Study the drawing (mm; zero at the part's minimum x, y, z) and answer. A direction names the side the tool comes from. Round coordinates to 2 decimals unless told otherwise and drop trailing zeros. Order: outer loops, then holes, each group sorted by start corner. A loop starts at its lowest first (then second) coordinate and runs counter-clockwise, first axis right, second up. Notation, with made-up numbers: (23.25, 50.25) - (46.25, 50.25) arc R23 cw to (46.25, 73.25) - close; hole circle Ø11 at (13, 67). An arc over 180 degrees is marked (long way). Put each result on its own line as item: value. Start each with the question number.
Q1. Each of these flat-tipped pins is pushed along its axis until it touches: pin 1 Ø3 at (x, z) = (9, 3) entering from +Y; pin 2 Ø3 at (x, z) = (13, 9.5) entering from -Y; pin 3 Ø1.5 at (y, z) = (1, 12.5) entering from -X; pin 4 Ø0.8 at (x, z) = (19.5, 18) entering from +Y. Where does it stop, or does it pass through?
Q2. Find the intervals of material crossed by line 1 along X through (y, z) = (6.9, 17.5) (3 decimals); line 2 along Z through (x, y) = (13.5, 3); line 3 along Y through (x, z) = (11, 12.5), in increasing order. Write a range as from..to.
Q3. Section C-C on z = 17.5 is taken. Give the vertices of the cut face in (x, y) (3 decimals), then the cut area to 3 significant figures.
Q4. Which of the six approach directions +Z, -Z, +X, -X, +Y, -Y give full straight-line access (tool end or side, diameter ignored) to the marked faces 5 and 6?
Q5. For a pull along Z with two mould halves and no side action, classify the marked faces 1, 2, 3 and 4 as pulls with the +Z half, pulls with the -Z half, needs draft (parallel to the pull), parting line crosses it, or undercut.
Q6. Section A-A on x = 19.45 is taken. Give the vertices of the cut face in (y, z) (3 decimals).
Q7. Section B-B on y = 4 is taken. Give the vertices of the cut face in (x, z).
Q8. Section D-D on x = 24.5 is taken. Give the vertices of the cut face in (y, z).
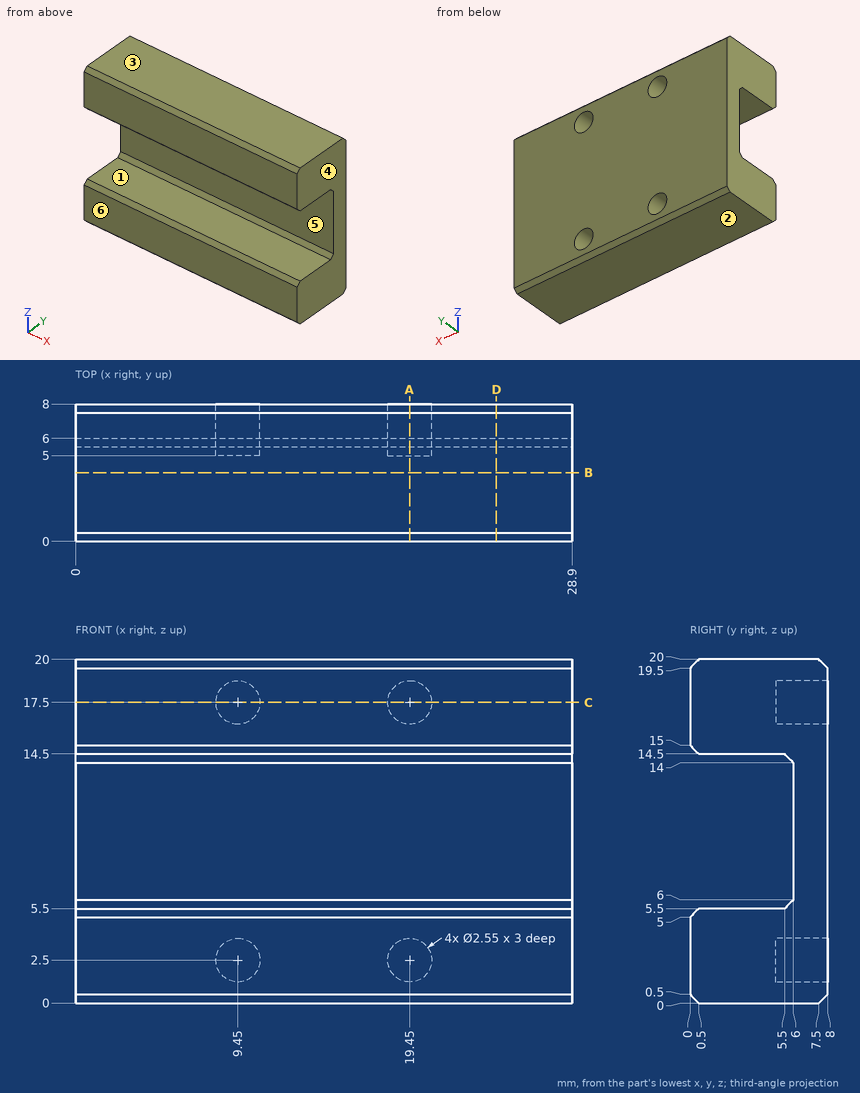
Findings:
1. pin 1: y = 8
1. pin 2: y = 6
1. pin 3: through
1. pin 4: y = 5
2. line 1: 0..8.175, 10.725..18.175, 20.725..28.9
2. line 2: 0..5.5, 14.5..20
2. line 3: 6..8
3. outline: (0, 0) - (28.9, 0) - (28.9, 8) - (20.725, 8) - (20.725, 5) - (18.175, 5) - (18.175, 8) - (10.725, 8) - (10.725, 5) - (8.175, 5) - (8.175, 8) - (0, 8) - close
3. area: 216 mm2
4. face 5: +X, -X, -Y
4. face 6: +Z, -Z, +X, -X, -Y
5. face 1: undercut
5. face 2: pulls with the -Z half
5. face 3: pulls with the +Z half
5. face 4: needs draft
6. outline: (0, 0.5) - (0.5, 0) - (7.5, 0) - (8, 0.5) - (8, 1.225) - (5, 1.225) - (5, 3.775) - (8, 3.775) - (8, 16.225) - (5, 16.225) - (5, 18.775) - (8, 18.775) - (8, 19.5) - (7.5, 20) - (0.5, 20) - (0, 19.5) - (0, 15) - (0.5, 14.5) - (5.5, 14.5) - (6, 14) - (6, 6) - (5.5, 5.5) - (0.5, 5.5) - (0, 5) - close
7. outline: (0, 0) - (28.9, 0) - (28.9, 5.5) - (0, 5.5) - close; (0, 14.5) - (28.9, 14.5) - (28.9, 20) - (0, 20) - close
8. outline: (0, 0.5) - (0.5, 0) - (7.5, 0) - (8, 0.5) - (8, 19.5) - (7.5, 20) - (0.5, 20) - (0, 19.5) - (0, 15) - (0.5, 14.5) - (5.5, 14.5) - (6, 14) - (6, 6) - (5.5, 5.5) - (0.5, 5.5) - (0, 5) - close
